from build123d import *

# Parameters (mm, degrees)
F0_W           = 120
F0_H           = 60
F1_DEPTH       = 90
F2_W           = 40
F2_H           = 70
F2_W_2         = 55
F3_DEPTH       = 60.001
F4_R           = 29.99999
F5_SIZE        = 8
F7_D           = 3.4
F7_CBORE_D     = 7
F7_CBORE_DEPTH = 2.4
F9_DEPTH       = 16
F11_DEPTH      = 60.001
F12_R          = 5


# Not quite as in the source:
# - a fillet or chamfer is up to 0.001 mm smaller than in the source, because OpenCascade refuses the exact size


with BuildPart() as f1:
    # F0 (on Top) → F1 (new body)
    with BuildSketch(Plane.XY):
        Rectangle(F0_W, F0_H)
    extrude(amount=F1_DEPTH)

    # F2 (on face) → F3 (cut, through all)
    with BuildSketch(Plane.XZ.offset(30)):
        with Locations((-40, 55)):
            Rectangle(F2_W, F2_H)
        with Locations((32.5, 55)):
            Rectangle(F2_W_2, F2_H)
    extrude(amount=-F3_DEPTH, mode=Mode.SUBTRACT)

    # F4 (radius 30 in the source; OpenCascade refuses exactly that, so slightly less here)
    f4_edges = [f1.edges().sort_by_distance(p)[0] for p in [
        (60, -30, 10),
        (60, 30, 10),
    ]]
    fillet(f4_edges, radius=F4_R)

    # F5
    f5_edges = [f1.edges().sort_by_distance(p)[0] for p in [
        (-60, -30, 10),
        (-60, 30, 10),
    ]]
    chamfer(f5_edges, length=F5_SIZE)

    # F7 (through all)
    with Locations(Plane(origin=(-20, 0, 0), x_dir=(0, -1, 0), z_dir=(-1, 0, 0))):
        with Locations((-20, 80), (20, 80), (20, 30), (-20, 30)):
            CounterBoreHole(F7_D / 2, F7_CBORE_D / 2, F7_CBORE_DEPTH)

    # F8 (on face) → F9 (cut)
    with BuildSketch(Plane.YZ.offset(5)):
        with BuildLine():
            ThreePointArc((10, 70), (0, 80), (-10, 70))
            ThreePointArc((-10, 70), (-7.0710678119, 62.9289321881), (0, 60))
            ThreePointArc((0, 60), (7.0710678119, 62.9289321881), (10, 70))
        make_face()
        with BuildLine():
            Line((10, 90), (-10, 90))
            Line((-10, 90), (-10, 70))
            ThreePointArc((-10, 70), (0, 80), (10, 70))
            Line((10, 70), (10, 90))
        make_face()
    extrude(amount=-F9_DEPTH, mode=Mode.SUBTRACT)

    # F10 (on face) → F11 (cut, through all)
    with BuildSketch(Plane.XZ.offset(30)):
        Polygon((5, 90), (-7.3428886496, 90), (5, 20), align=None)
    extrude(amount=-F11_DEPTH, mode=Mode.SUBTRACT)

    # F12
    f12_edges = [f1.edges().sort_by_distance(p)[0] for p in [
        (-13.671444, -30, 90),
        (-13.671444, 30, 90),
    ]]
    fillet(f12_edges, radius=F12_R)


solid = f1.part
Geometry check sheet. Reference: the model listing, model coordinates, mm. A direction names the side the tool comes from. Round coordinates to 2 decimals unless told otherwise and drop trailing zeros. Order: outer loops, then holes, each group sorted by start corner. A loop starts at its lowest first (then second) coordinate and runs counter-clockwise, first axis right, second up. Notation, with made-up numbers: M 39.25,83.25 L 83.25,83.25 A17 cw 83.25,89.25 Z; hole C 22,46.5 d4. An arc over 180 degrees is marked long. Answer in a Markdown table with one row per item. Add a question column.
Item 1: Sectioned sample at C-C, the plane z = 80. Enter the section's corners in (x, y).
Item 2: Set-up check for faces 1 (the face through (-20, 0, 55)), 2 (the face through (32, 0, 20)), 3 (the face through (-18.817, -19.241, 76.583)): record each of +Z, -Z, +X, -X, +Y, -Y from which the full face is reachable in a straight line by a thin tool's end or side.
Item 3: Draft check along Y on faces 4 (the face through (-11, 0, 75)), 5 (the face through (-17.6, 21, 28)), 6 (the face through (-1, 0, 0)), 7 (the face through (-12, -30, 23)). Enter one of: released by +Y, released by -Y, zero draft, split by the parting line, or undercut.
Item 4: Sectioned sample at B-B, the plane y = 20. Enter the section's corners in (x, z), plus the area to 3 significant figures.
Item 5: Sectioned sample at D-D, the plane y = 6. Enter the section's corners in (x, z).
Item 6: Depth check by flat-ended pin: pin 1 Ø9 at (y, z) = (-20, 30) entering from +X; pin 2 Ø5.5 at (y, z) = (20, 80) entering from +X; pin 3 Ø2 at (x, y) = (-43.5, -12) entering from +Z; pin 4 Ø2 at (y, z) = (-20, 30) entering from -X. Enter the tip coordinate at first touch or a pass-through.
Item 7: Material ranges on L1, parallel to Y at x = -12, z = 30; L2, parallel to Z at x = -18.35, y = 20; L3, parallel to Z at x = -8, y = -20, recorded low to high. Write a range as [from, to].
Filled in:
| question | item | result |
|---|---|---|
| 1 | outline | M -20,-30 L -5.58,-30 L -5.58,-21.7 L -17.6,-21.7 L -17.6,-23.5 L -20,-23.5 Z; M -20,-16.5 L -17.6,-16.5 L -17.6,-18.3 L -5.58,-18.3 L -5.58,-10 L -11,-10 L -11,10 L -5.58,10 L -5.58,18.3 L -17.6,18.3 L -17.6,16.5 L -20,16.5 Z; M -20,23.5 L -17.6,23.5 L -17.6,21.7 L -5.58,21.7 L -5.58,30 L -20,30 Z |
| 2 | face 1 | +Z, -X, +Y, -Y |
| 2 | face 2 | +Z, +X, +Y, -Y |
| 2 | face 3 | -X |
| 3 | face 4 | undercut |
| 3 | face 5 | undercut |
| 3 | face 6 | zero draft |
| 3 | face 7 | released by -Y |
| 4 | outline | M -60,0 L 52.36,0 L 52.36,20 L 5,20 L 3.54,28.3 L -17.6,28.3 L -17.6,26.5 L -20,26.5 L -20,20 L -60,20 Z; M -20,33.5 L -17.6,33.5 L -17.6,31.7 L 2.94,31.7 L -5.28,78.3 L -17.6,78.3 L -17.6,76.5 L -20,76.5 Z; M -20,83.5 L -17.6,83.5 L -17.6,81.7 L -5.88,81.7 L -7.34,90 L -20,90 Z |
| 4 | area | 3,420 mm² |
| 5 | outline | M -60,0 L 59.39,0 L 59.39,20 L 5,20 L -2.41,62 L -11,62 L -11,90 L -20,90 L -20,20 L -60,20 Z |
| 6 | pin 1 | stops at x = 4.03 |
| 6 | pin 2 | stops at x = -5.09 |
| 6 | pin 3 | stops at z = 20 |
| 6 | pin 4 | passes through |
| 7 | L1 | y = [-30, -21.7], [-18.3, 18.3], [21.7, 30] |
| 7 | L2 | z = [0, 26.5], [33.5, 76.5], [83.5, 90] |
| 7 | L3 | z = [0, 28.3], [31.7, 78.3], [81.7, 90] |
